Part model, mm, in its own coordinate system. A direction names the side the tool comes from. Give positions to 0.01 mm unless a question says otherwise; leave off trailing zeros. Order: outer loops, then holes, each group sorted by start corner. A loop starts at its lowest first (then second) coordinate and runs counter-clockwise, first axis right, second up. Notation, with made-up numbers: (26, 88.5) -> (75, 88.5) arc R30 cw to (75, 113.5) -> close; hole circle Ø1 at (-8, 10). An arc over 180 degrees is marked (long way). Write item = value, one per line. Start each with the question number.
(1) Saw through at A-A, the plane z = -5. List the corners of the cut face in (x, y), then the cut area to 3 significant figures.
(2) Saw through at D-D, the plane x = 70. List the corners of the cut face in (y, z), then the cut area to 3 significant figures.
(3) Probe line 1 along Y through (x, z) = (5, -5.25); line 2 along Y through (x, z) = (110, -7.5); line 3 along Z through (x, y) = (30, 5). List the from-to ranges inside material, lowest first. Write a range as from..to.
(4) Flat gauge pin, fed straight in: pin 1 (5 mm diameter, centred on y = 262.5, z = -2, fed in from -X). Where does the tip first touch, or does it go through?
(5) Saw through at C-C, the plane y = 93. List the corners of the cut face in (x, z), then the cut area to 3 significant figures.
(6) Saw through at B-B, the plane x = 89. List the corners of the cut face in (y, z).
(7) Which spindle directions (+Z, -Z, +X, -X, +Y, -Y) get a long thin tool onto all of the face, cutting with end or side? Do faces 1 (the cylindrical face through (71.23, 98.6, -4.56)), 2 (the flat face through (0, 153, -5)). Say none if no direction does.
Autodesk Inventor part; units mm, degrees
ref_plane "YZ Plane" through (0, 0, 0) normal (1, 0, 0) x (0, 1, 0)
ref_plane "XZ Plane" through (0, 0, 0) normal (0, 1, 0) x (-1, 0, 0)
ref_plane "XY Plane" through (0, 0, 0) normal (0, 0, 1) x (1, 0, 0)
sketch "Sketch1" plane through (0, 0, 0) normal (0, 1, 0) x (-1, 0, 0)
  line L0 (0, 0) -> (-80, 0)
  line L1 (-80, 0) -> (-80, -10)
  line L2 (-80, -10) -> (0, -10)
  line L3 (0, -10) -> (0, 0)
  arc A0 (-62.6378, -10) -> (-80, 0) centre (-130, -106.8831) ccw
  dimension "d1" = 10
  dimension "d2" = 118
  dimension "d3" = 80
  dimension "d4" = 50
extrude "Extrusion1" add sketch "Sketch1" along normal blind 200 contours L3 L2 A0 L0
sketch "Sketch4" plane through (0, 200, 0) normal (0, 1, 0) x (1, 0, 0)
  line L0 (0, 0) -> (130, 0)
  line L1 (130, 0) -> (130, 10)
  line L2 (130, 10) -> (0, 10)
  line L3 (0, 10) -> (0, 0)
  dimension "d24" = 130
  dimension "d25" = 10
sketch "Sketch3" plane through (0, 0, 0) normal (0, -1, 0) x (1, 0, 0)
  circle A0 centre (30, -5) radius 2
  line L0 (0, 0) -> (80, 0)
  line L1 (0, -10) -> (0, 0)
  dimension "d19" = 4
  dimension "d20" = 5
  dimension "d21" = 30
extrude "Extrusion3" cut sketch "Sketch3" against normal blind 20
sketch "Sketch2" plane through (0, 0, 0) normal (0, 0, 1) x (1, 0, 0)
  circle A0 centre (5, 30) radius 2
  line L0 (0, 0) -> (0, 200)
  line L1 (0, 0) -> (80, 0)
  circle A1 centre (5, 280) radius 2
  dimension "d7" = 4
  dimension "d8" = 5
  dimension "d9" = 30
  dimension "d12" = 250
extrude "Extrusion4" add sketch "Sketch4" along normal blind 110
extrude "Extrusion5" cut sketch "Sketch2" against normal through all
sketch "Sketch5" plane through (0, 0, 0) normal (0, 0, 1) x (1, 0, 0)
  circle A0 centre (110, 205) radius 2
  line L0 (130, 200) -> (130, 310)
  line L1 (80, 200) -> (130, 200)
  point P0 (0, 0)
  dimension "d30" = 4
  dimension "d31" = 20
  dimension "d32" = 5
extrude "Extrusion6" cut sketch "Sketch5" against normal through all
equation "\"d30\" = screws"
properties part number "box_front_left"
Results list:
q1.outline = (0, 0) -> (28, 0) -> (28, 20) -> (32, 20) -> (32, 0) -> (70.47, 0) -> (70.47, 200) -> (130, 200) -> (130, 310) -> (0, 310) -> close; hole circle Ø4 at (5, 30); hole circle Ø4 at (5, 280); hole circle Ø4 at (110, 205)
q1.area = 28,300 mm^2
q2.outline = (0, -5.28) -> (200, -5.28) -> (200, -10) -> (310, -10) -> (310, 0) -> (0, 0) -> close
q2.area = 2,160 mm^2
q3.line_1 = 0..28, 32..278, 282..310
q3.line_2 = 200..203, 207..310
q3.line_3 = -10..-7, -3..0
q4.pin_1 = 0
q5.outline = (0, -10) -> (62.64, -10) arc R118 cw to (80, 0) -> (0, 0) -> close
q5.area = 707 mm^2
q6.outline = (200, -10) -> (310, -10) -> (310, 0) -> (200, 0) -> close
q7.face_1 = -Z, +X, -Y
q7.face_2 = +Z, -Z, -X, +Y, -Y
